Autodesk Inventor part; units mm, degrees
ref_plane "YZ Plane" through (0, 0, 0) normal (1, 0, 0) x (0, 1, 0)
ref_plane "XZ Plane" through (0, 0, 0) normal (0, 1, 0) x (-1, 0, 0)
ref_plane "XY Plane" through (0, 0, 0) normal (0, 0, 1) x (1, 0, 0)
sketch "Sketch1" plane through (0, 0, 0) normal (0, 0, 1) x (1, 0, 0)
  circle A0 centre (0, 0) radius 9.625
  arc A1 (0, 12.5) -> (0, -12.5) centre (0, 0) ccw
  line L0 (0, -12.5) -> (37.5, -12.5)
  line L1 (37.5, -12.5) -> (37.5, 12.5)
  line L2 (37.5, 12.5) -> (0, 12.5)
  line L3 (37.5, 0) -> (9.625, 0) construction
  dimension "d0" = 19.25
  dimension "d2" = 25
  dimension "d4" = 37.5
extrude "Extrusion1" add sketch "Sketch1" along normal blind 25
sketch "Sketch2" plane through (0, -12.5, 0) normal (0, -1, 0) x (1, 0, 0)
  line L0 (37.5, 0) -> (37.5, 25)
  line L1 (0, 25) -> (37.5, 25)
  line L2 (0, 0) -> (0, 25)
  line L3 (37.5, 0) -> (50, 0)
  line L4 (50, 0) -> (50, 12.5)
  arc A0 (50, 12.5) -> (37.5, 25) centre (37.5, 12.5) ccw
extrude "Extrusion2" add sketch "Sketch2" against normal up to surface (25 mm away)
sketch "Sketch3" plane through (0, -12.5, 0) normal (0, -1, 0) x (1, 0, 0)
  arc A0 (50, 12.5) -> (37.5, 25) centre (37.5, 12.5) ccw
  circle A1 centre (37.5, 12.5) radius 4.1
  dimension "d9" = 8.2
extrude "Extrusion3" cut sketch "Sketch3" against normal through all
sketch "Sketch10" plane through (50, 12.5, 12.5) normal (0, 1, 0) x (1, 0, 0)
  circle A0 centre (-12.5, 0) radius 4.1
  line L0 (-20.121, 0) -> (-16.3105, 6.6)
  line L1 (-16.3105, 6.6) -> (-8.6895, 6.6)
  line L2 (-8.6895, 6.6) -> (-4.879, 0)
  line L3 (-4.879, 0) -> (-8.6895, -6.6)
  line L4 (-8.6895, -6.6) -> (-16.3105, -6.6)
  line L5 (-16.3105, -6.6) -> (-20.121, 0)
  point P0 (-50, 12.5)
  point P1 (-12.5, 6.6)
  dimension "d47" = 13.2
extrude "Extrusion10" cut sketch "Sketch10" against normal blind 8
sketch "Sketch11" plane through (0, 0, 0) normal (0, 0, -1) x (-1, 0, 0)
  circle A0 centre (0, 0) radius 9.625
  arc A1 (0, -12.5) -> (0, 12.5) centre (0, 0) ccw
  circle A2 centre (0, 0) radius 19.05
  dimension "d50" = 38.1
extrude "Extrusion11" add sketch "Sketch11" against normal up to surface (25 mm away)
sketch "Sketch12" plane through (0, 0, 0) normal (0, 0, -1) x (-1, 0, 0)
  arc A0 (-14.3754, -12.5) -> (-14.3754, 12.5) centre (0, 0) ccw
  circle A1 centre (14.2875, 0) radius 1.6
  dimension "d55" = 14.2875
  dimension "d56" = 3.2
extrude "Extrusion12" cut sketch "Sketch12" against normal through all
sketch "Sketch13" plane through (0, 0, 25) normal (0, 0, 1) x (1, 0, 0)
  circle A0 centre (-14.2875, 0) radius 1.6
  line L0 (-14.2875, 3.262) -> (-11.4625, 1.631)
  line L1 (-11.4625, 1.631) -> (-11.4625, -1.631)
  line L2 (-11.4625, -1.631) -> (-14.2875, -3.262)
  line L3 (-14.2875, -3.262) -> (-17.1125, -1.631)
  line L4 (-17.1125, -1.631) -> (-17.1125, 1.631)
  line L5 (-17.1125, 1.631) -> (-14.2875, 3.262)
  dimension "d59" = 5.65
extrude "Extrusion13" cut sketch "Sketch13" against normal blind 3
pattern_circular "Circular Pattern3" count 3 over 360 about axis through (0, 0, 0) along (0, 0, 1) of "Extrusion13", "Extrusion12"
properties part number "SHOULDER"
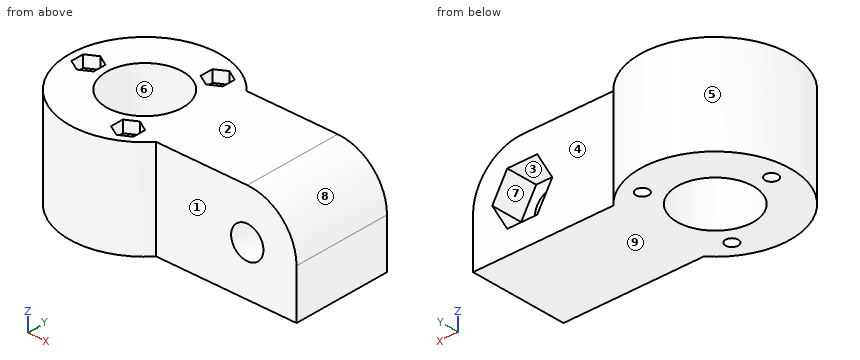
Geometry: final body of the model. Coordinates: model frame, mm. Face numbers are marked on the shaded views. A direction names the side the tool comes from. Round coordinates to 2 decimals unless told otherwise and drop trailing zeros. Order: outer loops, then holes, each group sorted by start corner. A loop starts at its lowest first (then second) coordinate and runs counter-clockwise, first axis right, second up. Notation, with made-up numbers: (-18.5, 81) -> (18.5, 81) arc R13 ccw to (18.5, 100) -> close; hole circle Ø11 at (-40, -36.75). An arc over 180 degrees is marked (long way). Use one line per item in the form item = value.
(1) Ray query, probe 1 along X at (y, z) = (6.5, 10.5); probe 2 along X at (y, z) = (-4.5, 13.25); probe 3 along Y at (x, z) = (0, 5) (3 decimals). Return the intervals inside material, ascending. Write a range as [from, to].
Results list:
probe_1 = [-17.91, -7.1], [7.1, 31.03], [43.97, 50]
probe_2 = [-18.51, -8.51], [8.51, 33.47], [41.53, 49.98]
probe_3 = [-19.05, -9.625], [9.625, 19.05]
(2) First-contact query: pin 1 Ø1.5 at (x, z) = (10.5, 18) entering from +Y; pin 2 Ø2.5 at (y, z) = (12, 23.5) entering from +X; pin 3 Ø6 at (x, z) = (12.5, 13.5) entering from +Y. Flat tips, straight axial feed; report the tip coordinate or a pass-through.
Results list:
pin_1 = 16.37
pin_2 = 45.32
pin_3 = 16.51
(3) Draft query along Z for the marked faces 6, 7, 8 and 9. Return one class per face: pulls with the +Z half, pulls with the -Z half, needs draft (parallel to the pull), parting line crosses it, or undercut.
Results list:
face_6 = needs draft
face_7 = undercut
face_8 = pulls with the +Z half
face_9 = pulls with the -Z half
(4) Section D-D on y = 7. Return loops of the section in (x, z), and give its area (3 significant figures).
Results list:
outline = (-17.72, 0) -> (-6.61, 0) -> (-6.61, 25) -> (-17.72, 25) -> close; (6.61, 0) -> (50, 0) -> (50, 12.5) arc R12.5 ccw to (37.5, 25) -> (6.61, 25) -> close; hole (29.88, 12.5) -> (33.69, 5.9) -> (41.31, 5.9) -> (45.12, 12.5) -> (41.31, 19.1) -> (33.69, 19.1) -> close
area = 1,180 mm^2
(5) Section A-A on y = 0. Count the separate pieces of the cut face and the enclosed holes in it, and give its area (3 significant figures).
Results list:
separate_pieces = 3
enclosed_holes = 1
area = 1,070 mm^2
(6) Access query for the marked faces 1, 2, 3, 4 and 5. Directions: +Z, -Z, +X, -X, +Y, -Y. A direction counts if a zero-diameter tool reaches every point of the face in a straight line with its end or side. Return the directions, or none.
Results list:
face_1 = +Z, -Z, +X, -Y
face_2 = +Z, +X, -X, +Y, -Y
face_3 = +Y
face_4 = +Z, -Z, +X, +Y
face_5 = +Z, -Z
(7) Section B-B on x = 0. Return loops of the section in (y, z) (3 decimals), and give its area (3 significant figures).
Results list:
outline = (-19.05, 0) -> (-9.625, 0) -> (-9.625, 25) -> (-19.05, 25) -> close; (9.625, 0) -> (19.05, 0) -> (19.05, 25) -> (9.625, 25) -> close
area = 471 mm^2
